```python
from build123d import *

# Parameters (mm, degrees)
BOSS_EXTRUDE1_DEPTH      = 1
BOSS_EXTRUDE2_DEPTH      = 11
BOSS_EXTRUDE3_DEPTH      = 5
BOSS_EXTRUDE3_DEPTH_BACK = 3
SKETCH3_W                = 50
SKETCH3_H                = 7
CUT_EXTRUDE3_DEPTH       = 25
SKETCH5_W                = 50
SKETCH5_H                = 7
CUT_EXTRUDE4_DEPTH       = 25
SKETCH6_W                = 50
SKETCH6_H                = 7
CUT_EXTRUDE5_DEPTH       = 25
SKETCH8_R                = 1.5
BOSS_EXTRUDE5_DEPTH      = 1
BOSS_EXTRUDE10_DEPTH     = 5.5


with BuildPart() as part:
    # Sketch1 → Boss-Extrude1 (new body)
    with BuildSketch(Plane(origin=(0, 0, 0), x_dir=(1, 0, 0), z_dir=(0, 1, 0))):
        Polygon((243.304219773, -116.484791866), (254.809280576, -136.408896139), (442.602090749, -136.409305398), (444.621046679, -132.925433223), (441.749040748, -132.925433223), (449.516726723, -119.471406457), (450.964695297, -121.978953122), (452.699916621, -118.984688017), (358.778179035, 43.666038066), (335.767496284, 43.666038066), align=None)
        Polygon((428.113670919, -116.417164681), (266.439108268, -116.428009241), (347.273609729, 23.609230825), align=None, mode=Mode.SUBTRACT)
    extrude(amount=BOSS_EXTRUDE1_DEPTH)

    # Sketch1_9 → Boss-Extrude2 (add)
    # profile 1 of 2: a face of its own
    with BuildSketch(Plane(origin=(0, 0, 0), x_dir=(1, 0, 0), z_dir=(0, 1, 0))):
        Polygon((229.159432547, -134.984249184), (231.716666588, -139.412373829), (462.829865412, -139.412373829), (465.38624875, -134.984588004), (349.829542096, 65.165499075), (344.716133219, 65.165499075), align=None)
        Polygon((251.922647988, -136.4093054), (233.446303399, -136.408896139), (232.623553959, -134.984217358), (241.860901688, -118.984688019), align=None, mode=Mode.SUBTRACT)
        Polygon((442.602090749, -136.409305398), (254.809280576, -136.408896139), (243.304219773, -116.484791866), (335.767496284, 43.666038066), (358.778179035, 43.666038066), (461.938967957, -134.984588004), (461.116393748, -136.409305398), align=None, mode=Mode.SUBTRACT)
        Polygon((348.096628302, 62.164013367), (357.334800991, 46.166038067), (337.210874326, 46.166038067), (346.44844193, 62.165948237), align=None, mode=Mode.SUBTRACT)
    # profile 2 of 2: a face of its own
    with BuildSketch(Plane(origin=(0, 0, 0), x_dir=(1, 0, 0), z_dir=(0, 1, 0))):
        Polygon((441.749040748, -132.925433223), (444.621046679, -132.925433223), (450.964695297, -121.978953122), (449.516726723, -119.471406457), align=None)
    extrude(amount=BOSS_EXTRUDE2_DEPTH)

    # Sketch1_10 → Boss-Extrude3 (add, two sides: drawn at the far end of the back side and taken through both)
    with BuildSketch(Plane(origin=(0, 0, 0), x_dir=(1, 0, 0), z_dir=(0, 1, 0)).offset(-BOSS_EXTRUDE3_DEPTH_BACK)):
        Polygon((229.159432547, -134.984249184), (231.716666588, -139.412373829), (462.829865412, -139.412373829), (465.38624875, -134.984588004), (349.829542096, 65.165499075), (344.716133219, 65.165499075), align=None)
        Polygon((251.922647988, -136.4093054), (233.446303399, -136.408896139), (232.623553959, -134.984217358), (241.860901688, -118.984688019), align=None, mode=Mode.SUBTRACT)
        Polygon((442.602090749, -136.409305398), (254.809280576, -136.408896139), (243.304219773, -116.484791866), (335.767496284, 43.666038066), (358.778179035, 43.666038066), (452.699916621, -118.984688017), (461.938967957, -134.984588004), (461.116393748, -136.409305398), align=None, mode=Mode.SUBTRACT)
        Polygon((348.096628302, 62.164013367), (357.334800991, 46.166038067), (337.210874326, 46.166038067), (346.44844193, 62.165948237), align=None, mode=Mode.SUBTRACT)
    extrude(amount=BOSS_EXTRUDE3_DEPTH + BOSS_EXTRUDE3_DEPTH_BACK)

    # Sketch3 → Cut-Extrude3 (cut)
    with BuildSketch(Plane(origin=(290.589645397, 0, -167.772009994), x_dir=(-0.49999999999998745, 0, -0.8660254037844459), z_dir=(0.8660254037844459, 0, -0.49999999999998745))):
        with Locations((-236.592990632, -3)):
            Rectangle(SKETCH3_W, SKETCH3_H)
    extrude(amount=-CUT_EXTRUDE3_DEPTH, mode=Mode.SUBTRACT)

    # Sketch5 → Cut-Extrude4 (cut)
    with BuildSketch(Plane.XY.offset(139.412373829)):
        with Locations((347.273266, -3)):
            Rectangle(SKETCH5_W, SKETCH5_H)
    extrude(amount=-CUT_EXTRUDE4_DEPTH, mode=Mode.SUBTRACT)

    # Sketch6 → Cut-Extrude5 (cut)
    with BuildSketch(Plane(origin=(230.319375797, 0, 132.975171838), x_dir=(-0.5000006154012504, 0, 0.8660250484820695), z_dir=(-0.8660250484820695, 0, -0.5000006154012504))):
        with Locations((-113.2366748, -3)):
            Rectangle(SKETCH6_W, SKETCH6_H)
    extrude(amount=-CUT_EXTRUDE5_DEPTH, mode=Mode.SUBTRACT)

    # Sketch8 → Boss-Extrude5 (add)
    with BuildSketch(Plane.XZ.offset(3)):
        Polygon((246.891774838, 127.696996709), (240.128710529, 115.984933576), (333.74677129, -46.166038067), (360.798886024, -46.166038067), (454.427535986, 116.00354071), (450.14703547, 123.280701064), (406.618322212, 98.678849058), (401.697951811, 107.384591709), (445.226665069, 131.986443715), (440.912417704, 139.412373829), (253.656752788, 139.412373829), align=None)
        with Locations(Location((395.323540807, 98.692824234, 0), (0, 0, 270))):
            Circle(SKETCH8_R, mode=Mode.SUBTRACT)
        with Locations(Location((348.301285092, 15.863526629, 0), (0, 0, 270))):
            Circle(SKETCH8_R, mode=Mode.SUBTRACT)
        with Locations(Location((299.654911442, 97.241681781, 0), (0, 0, 270))):
            Circle(SKETCH8_R, mode=Mode.SUBTRACT)
        Polygon((322.273266, 116.424264082), (294.358218631, 68.061097964), (319.354499366, 24.757680453), (376.473657317, 26.969372805), (401.47267951, 70.271207531), (372.273266, 116.420910258), align=None, mode=Mode.SUBTRACT)
    extrude(amount=BOSS_EXTRUDE5_DEPTH)

    # Sketch12 → Boss-Extrude10 (add)
    with BuildSketch(Plane(origin=(0, -3, 0), x_dir=(1, 0, 0), z_dir=(0, 1, 0))):
        with BuildLine():
            Line((347.417900212, -11.962292061), (347.307477102, -11.47463774))
            ThreePointArc((347.307477102, -11.47463774), (345.119304576, -12.681546113), (343.912396203, -14.869718639))
            Line((343.912396203, -14.869718639), (344.400050524, -14.980141749))
            ThreePointArc((344.400050524, -14.980141749), (345.472857967, -13.035099504), (347.417900212, -11.962292061))
        make_face()
        with BuildLine():
            ThreePointArc((352.69017398, -14.869718639), (351.483265607, -12.681546113), (349.295093082, -11.47463774))
            Line((349.295093082, -11.47463774), (349.184669972, -11.962292061))
            ThreePointArc((349.184669972, -11.962292061), (351.129712216, -13.035099504), (352.202519659, -14.980141749))
            Line((352.202519659, -14.980141749), (352.69017398, -14.869718639))
        make_face()
        with BuildLine():
            ThreePointArc((349.295093082, -20.252415518), (351.483265607, -19.045507144), (352.69017398, -16.857334619))
            Line((352.69017398, -16.857334619), (352.202519659, -16.746911509))
            ThreePointArc((352.202519659, -16.746911509), (351.129712216, -18.691953754), (349.184669972, -19.764761197))
            Line((349.184669972, -19.764761197), (349.295093082, -20.252415518))
        make_face()
        with BuildLine():
            Line((344.400050524, -16.746911509), (343.912396203, -16.857334619))
            ThreePointArc((343.912396203, -16.857334619), (345.119304576, -19.045507144), (347.307477102, -20.252415518))
            Line((347.307477102, -20.252415518), (347.417900212, -19.764761197))
            ThreePointArc((347.417900212, -19.764761197), (345.472857967, -18.691953754), (344.400050524, -16.746911509))
        make_face()
        with BuildLine():
            Line((394.440155927, -94.791589666), (394.329732817, -94.303935345))
            ThreePointArc((394.329732817, -94.303935345), (392.141560292, -95.510843719), (390.934651919, -97.699016244))
            Line((390.934651919, -97.699016244), (391.4247896, -97.798542945))
            ThreePointArc((391.4247896, -97.798542945), (392.499067689, -95.860448622), (394.440155927, -94.791589666))
        make_face()
        with BuildLine():
            ThreePointArc((399.712429696, -97.699016244), (398.505521323, -95.510843719), (396.317348797, -94.303935345))
            Line((396.317348797, -94.303935345), (396.206925687, -94.791589666))
            ThreePointArc((396.206925687, -94.791589666), (398.151967932, -95.864397109), (399.224775375, -97.809439354))
            Line((399.224775375, -97.809439354), (399.712429696, -97.699016244))
        make_face()
        with BuildLine():
            ThreePointArc((396.317348797, -103.081713123), (398.505521323, -101.874804749), (399.712429696, -99.686632224))
            Line((399.712429696, -99.686632224), (399.224775375, -99.576209114))
            ThreePointArc((399.224775375, -99.576209114), (398.151967932, -101.521251359), (396.206925687, -102.594058802))
            Line((396.206925687, -102.594058802), (396.317348797, -103.081713123))
        make_face()
        with BuildLine():
            Line((391.422306239, -99.576209114), (390.934651919, -99.686632224))
            ThreePointArc((390.934651919, -99.686632224), (392.141560292, -101.874804749), (394.329732817, -103.081713123))
            Line((394.329732817, -103.081713123), (394.440155927, -102.594058802))
            ThreePointArc((394.440155927, -102.594058802), (392.495113683, -101.521251359), (391.422306239, -99.576209114))
        make_face()
        with BuildLine():
            ThreePointArc((298.661103452, -92.852792892), (296.472930927, -94.059701266), (295.266022553, -96.247873791))
            Line((295.266022553, -96.247873791), (295.753676874, -96.358296901))
            ThreePointArc((295.753676874, -96.358296901), (296.826484317, -94.413254657), (298.771526562, -93.340447213))
            Line((298.771526562, -93.340447213), (298.661103452, -92.852792892))
        make_face()
        with BuildLine():
            ThreePointArc((304.043800331, -96.247873791), (302.836891957, -94.059701266), (300.648719432, -92.852792892))
            Line((300.648719432, -92.852792892), (300.538296322, -93.340447213))
            ThreePointArc((300.538296322, -93.340447213), (302.483338567, -94.413254657), (303.55614601, -96.358296901))
            Line((303.55614601, -96.358296901), (304.043800331, -96.247873791))
        make_face()
        with BuildLine():
            Line((300.538296322, -101.142916349), (300.648719432, -101.63057067))
            ThreePointArc((300.648719432, -101.63057067), (302.836891957, -100.423662297), (304.043800331, -98.235489771))
            Line((304.043800331, -98.235489771), (303.55614601, -98.125066661))
            ThreePointArc((303.55614601, -98.125066661), (302.483338567, -100.070108906), (300.538296322, -101.142916349))
        make_face()
        with BuildLine():
            Line((295.753676874, -98.125066661), (295.266022553, -98.235489771))
            ThreePointArc((295.266022553, -98.235489771), (296.472930927, -100.423662297), (298.661103452, -101.63057067))
            Line((298.661103452, -101.63057067), (298.771526562, -101.142916349))
            ThreePointArc((298.771526562, -101.142916349), (296.826484317, -100.070108906), (295.753676874, -98.125066661))
        make_face()
    extrude(amount=BOSS_EXTRUDE10_DEPTH)


solid = part.part
```
Can you work these out from the model? Positions are in its coordinate system, mm. A direction names the side the tool comes from. Give positions to 0.01 mm unless a question says otherwise; leave off trailing zeros. Order: outer loops, then holes, each group sorted by start corner. A loop starts at its lowest first (then second) coordinate and runs counter-clockwise, first axis right, second up. Notation, with made-up numbers: M 5.25,80.5 L 40.25,80.5 A17 cw 40.25,96.5 Z; hole C -30,-1.75 d8. An arc over 180 degrees is marked long. Write item = value, one per line. Start each with the question number.
Q1. Will these pins go through, and if not, where does the flat tip stop? pin 1 Ø6 at (x, y) = (285.5, 0) entering from -Z; pin 2 Ø1.8 at (x, z) = (297, 95) entering from +Y; pin 3 Ø6 at (y, z) = (4.5, 19) entering from +X.
Q2. Suppose I cut it at B-B (z = -36). Write out the boundary of the cut face in (x, y), plus the area to 3 significant figures.
Q3. For faces 1 (the flat face through (297, 0.5, 40)), 2 (the flat face through (235, -3, 130)), 3 (the flat face through (347, 6, -43.666)), 4 (the flat face through (423.158, -3.493, 119.513)), 5 (the flat face through (351, -3, -58)), which set-ups out of +Z, -Z, +X, -X, +Y, -Y let a thin tool reach every point of the face, with its end or its side?
Q4. Suppose I cut it at C-C (x = 384.5). Write out the boundary of the cut face in (y, z).
Q5. Suppose I cut it at A-A (y = 6.75). Write out the boundary of the cut face in (x, z), plus the area to 3 significant figures.
Q6. Suppose I cut it at D-D (x = 270.5). Write out the boundary of the cut face in (y, z), plus the area to 3 significant figures.
Q7. We'd pull the mould along X, two halves only. Please class faces 6 (the flat face through (298, -4, 89)), 7 (the flat face through (318.666, -1.521, -14.045)): pulls with the +X half, pulls with the -X half, needs draft (parallel to the pull), parting line crosses it, or undercut.
Q8. I need wall thicknesses on probe 1 along Y at (x, z) = (422, 123); probe 2 along Y at (x, z) = (292, 47.5); probe 3 along Z at (x, y) = (248, -1.5). Which ranges of each line are inside material? Lowest first, please. Write a range as [from, to].
Check result:
q1.pin_1 = 32.28
q1.pin_2 = 2.5
q1.pin_3 = 400.15
q2.outline = M 327.88,-4 L 366.67,-4 L 366.67,11 L 363.2,11 L 363.2,1 L 331.34,1 L 331.34,11 L 327.88,11 Z; hole M 331.34,-3 L 363.2,-3 L 363.2,0 L 331.34,0 Z
q2.area = 168 mm2
q3.face_1 = none
q3.face_2 = +Z, -X, -Y
q3.face_3 = +Y
q3.face_4 = -Y
q3.face_5 = -Z, +X, -X, -Y
q4.outline = M -4,-5.11 L 11,-5.11 L 11,0.88 L 1,0.88 L 1,40.87 L 0.5,40.87 L 0.5,22.34 L 0,22.34 L 0,0.88 L -3,0.88 L -3,40.87 L -4,40.87 Z; M -4,97.1 L -3,97.1 L -3,136.41 L 0,136.41 L 0,116.42 L 1,116.42 L 1,136.41 L 11,136.41 L 11,139.41 L -4,139.41 Z
q5.outline = M 229.16,134.98 L 344.72,-65.17 L 349.83,-65.17 L 465.39,134.98 L 462.83,139.41 L 231.72,139.41 Z; M 441.75,132.93 L 449.52,119.47 L 450.96,121.98 L 444.62,132.93 Z; hole M 232.62,134.98 L 241.86,118.98 L 251.92,136.41 L 233.45,136.41 Z; hole M 243.3,116.48 L 335.77,-43.67 L 358.78,-43.67 L 461.94,134.98 L 461.12,136.41 L 442.6,136.41 L 254.81,136.41 Z; hole M 337.21,-46.17 L 346.45,-62.17 L 348.1,-62.16 L 357.33,-46.17 Z
q5.area = 2,240 mm2
q6.outline = M -4,63.38 L 11,63.38 L 11,69.38 L 1,69.38 L 1,109.39 L 0,109.39 L 0,69.38 L -3,69.38 L -3,136.41 L 0,136.41 L 0,116.43 L 1,116.43 L 1,136.41 L 11,136.41 L 11,139.41 L -4,139.41 Z
q6.area = 262 mm2
q7.face_6 = needs draft
q7.face_7 = undercut
q8.probe_1 = [-4, -3], [0, 1]
q8.probe_2 = [-4, -3], [0.5, 1]
q8.probe_3 = [102.35, 108.35], [124.62, 129.62], [136.41, 139.41]
